Autodesk Inventor part; units mm, degrees
ref_plane "YZ Plane" through (0, 0, 0) normal (1, 0, 0) x (0, 1, 0)
ref_plane "XZ Plane" through (0, 0, 0) normal (0, 1, 0) x (-1, 0, 0)
ref_plane "XY Plane" through (0, 0, 0) normal (0, 0, 1) x (1, 0, 0)
sketch "Sketch2" plane through (0, 0, 0) normal (0, 1, 0) x (-1, 0, 0)
  line L0 (-44.45, 50.8) -> (44.45, 50.8)
  line L1 (44.45, 50.8) -> (44.45, -50.8)
  line L2 (44.45, -50.8) -> (-44.45, -50.8)
  line L3 (-44.45, -50.8) -> (-44.45, 50.8)
  point P0 (0, 0)
  dimension "d0" = 44.45
  dimension "d1" = 44.45
  dimension "d2" = 50.8
  dimension "d3" = 50.8
extrude "Extrusion1" add sketch "Sketch2" along normal blind 3.175
fillet "Fillet1" radius 12.7 4 edges at (44.45, 1.5875, 50.8) (-44.45, 1.5875, 50.8) (44.45, 1.5875, -50.8) (-44.45, 1.5875, -50.8)
sketch "Sketch3" plane through (0, 3.175, 0) normal (0, 1, 0) x (1, 0, 0)
  line L0 (-19.05, 38.1) -> (19.05, 38.1) construction
  line L1 (19.05, 38.1) -> (19.05, -38.1) construction
  line L2 (19.05, -38.1) -> (-19.05, -38.1) construction
  line L3 (-19.05, -38.1) -> (-19.05, 38.1) construction
  point P0 (0, 0)
  point P1 (0, 0)
  point P2 (-19.05, 0)
  point P3 (0, 38.1)
  dimension "d36" = 38.1
  dimension "d37" = 76.2
hole "Hole1" at (-19.05, 3.175, -38.1) at (19.05, 3.175, -38.1) at (19.05, 3.175, 38.1) at (-19.05, 3.175, 38.1) at (0, 3.175, 0) direction (0, -1, 0) diameter 6.35 end through all
sketch "Sketch4" plane through (0, 0, 0) normal (0, -1, 0) x (1, 0, 0)
  circle A0 centre (-19.05, 38.1) radius 3.175
  line L0 (44.45, -38.1) -> (44.45, 38.1)
  line L1 (-44.45, 38.1) -> (-44.45, -38.1)
  line L2 (44.45, 38.1) -> (41.275, 38.1)
  line L3 (41.275, 38.1) -> (41.275, -38.1)
  line L4 (41.275, -38.1) -> (44.45, -38.1)
  line L5 (44.45, -38.1) -> (44.45, 38.1)
  line L6 (-44.45, 38.1) -> (-41.275, 38.1)
  line L7 (-41.275, 38.1) -> (-41.275, -38.1)
  line L8 (-41.275, -38.1) -> (-44.45, -38.1)
  line L9 (-44.45, -38.1) -> (-44.45, 38.1)
  dimension "d18" = 3.175
  dimension "d19" = 3.175
  dimension "d20" = 76.2
  dimension "d21" = 76.2
extrude "Extrusion2" add sketch "Sketch4" along normal blind 95.25 contours L4 L3 L2 L0 | L6 L7 L8 L1
sketch "Sketch5" plane through (44.45, 3.175, 38.1) normal (1, 0, 0) x (0, 0, -1)
  line L0 (0, -3.175) -> (0, -98.425)
  line L1 (76.2, -3.175) -> (76.2, -98.425)
  line L2 (0, -3.175) -> (25.4, -98.425)
  line L3 (76.2, -3.175) -> (50.8, -98.425)
  line L4 (0, -3.175) -> (0, -98.425)
  line L5 (25.4, -98.425) -> (0, -98.425)
  line L6 (50.8, -98.425) -> (76.2, -98.425)
  line L7 (76.2, -98.425) -> (76.2, -3.175)
  point P0 (38.1, -3.175)
extrude "Extrusion3" cut sketch "Sketch5" against normal blind 127
sketch "Sketch6" plane through (44.45, 3.175, 38.1) normal (1, 0, 0) x (0, 0, -1)
  line L0 (25.4, -98.425) -> (50.8, -98.425)
  point P0 (38.1, -3.175)
  point P1 (38.1, -88.9)
  dimension "d28" = 9.525
hole "Hole2" at (44.45, -85.725, 0) direction (-1, 0, 0) diameter 12.7 end through all
equation "\"d4\" = metalThickness"
equation "\"d18\" = metalThickness"
equation "\"d19\" = metalThickness"
equation "\"d21\" = d20"
equation "\"metalThickness\" = 3.175"
properties part number "Caster2" material "Aluminum-6061"
Design review of the part built by this model. Coordinates are the model's own, in mm. A direction names the side the tool comes from. Coordinates: 2 decimals unless noted, no trailing zeros. Write each loop counter-clockwise with the first axis right and the second up, starting at its lowest first coordinate (ties: lowest second). Pieces come first, ordered by that corner, then holes.
1) Add section A-A (x = 0). Write out the cut boundary in (y, z) (3 decimals).
2) Add section B-B (y = -42). Write out the cut boundary in (x, z) (3 decimals), plus the area to 3 significant figures.
3) Insertion check: pin 1 (1.5 mm diameter, centred on x = 15.5, z = 10.5, fed in from -Y). The pin has a flat end and moves straight along its axis. Give the tip position at first contact, or say it passes through.
4) Machinability: for faces 1 (the flat face through (-41.275, -36, 1)), 2 (the flat face through (11, 3.175, 1)), which of the approach directions +Z, -Z, +X, -X, +Y, -Y give a long, thin tool a straight path to every point of the face, cutting with its end or side? Answer none if there is none.
5) Add section D-D (z = 0). Write out the cut boundary in (x, y) (3 decimals).
6) To check wall thickness, follow L1, parallel to Z at x = -19.05, y = 2.1 (3 decimals); L2, parallel to X at y = 1, z = 38; L3, parallel to X at y = -13.5, z = 29 (3 decimals). State the ranges of each line that lie inside material, in increasing order.
7) Add section C-C (x = 19.05). Write out the cut boundary in (y, z) (3 decimals), plus the area to 3 significant figures.
8) Mouldability with a two-part tool opening along X and no side actions: class faces 3 (the cylindrical face through (-40.83, 1.61, 46.98)), 4 (the cylindrical face through (18.91, 1.57, -41.27)), 5 (the flat face through (0, 2, 50.8)), 6 (the flat face through (41.275, -36, 1)) as +X half, -X half, draft (parallel to the pull), parting line (faces both ways), or undercut.
Check result:
1. outline: (0, -50.8) - (3.175, -50.8) - (3.175, -3.175) - (0, -3.175) - close; (0, 3.175) - (3.175, 3.175) - (3.175, 50.8) - (0, 50.8) - close
2. outline: (-44.45, -26.9) - (-41.275, -26.9) - (-41.275, 26.9) - (-44.45, 26.9) - close; (41.275, -26.9) - (44.45, -26.9) - (44.45, 26.9) - (41.275, 26.9) - close
2. area: 342 mm2
3. pin 1: stops at y = 0
4. face 1: +Z, -Z, -Y
4. face 2: +Z, -Z, +X, -X, +Y
5. outline: (-44.45, -95.25) - (-41.275, -95.25) - (-41.275, -92.075) - (-44.45, -92.075) - close; (-44.45, -79.375) - (-41.275, -79.375) - (-41.275, 0) - (-3.175, 0) - (-3.175, 3.175) - (-44.45, 3.175) - close; (3.175, 0) - (41.275, 0) - (41.275, -79.375) - (44.45, -79.375) - (44.45, 3.175) - (3.175, 3.175) - close; (41.275, -95.25) - (44.45, -95.25) - (44.45, -92.075) - (41.275, -92.075) - close
6. L1: z = -50.8 to -41.275, -34.925 to 34.925, 41.275 to 50.8
6. L2: x = -44.45 to -22.22, -15.88 to 15.88, 22.22 to 44.45
6. L3: x = -44.45 to -41.275, 41.275 to 44.45
7. outline: (0, -50.8) - (3.175, -50.8) - (3.175, -41.275) - (0, -41.275) - close; (0, -34.925) - (3.175, -34.925) - (3.175, 34.925) - (0, 34.925) - close; (0, 41.275) - (3.175, 41.275) - (3.175, 50.8) - (0, 50.8) - close
7. area: 282 mm2
8. face 3: -X half
8. face 4: undercut
8. face 5: draft
8. face 6: undercut
